```python
from build123d import *
from build123d.topology import SkipClean

# Parameters (mm, degrees)
BOSS_EXTRUDE1_DEPTH = 6
BOSS_EXTRUDE2_START = 6
SKETCH3_R           = 13
BOSS_EXTRUDE2_DEPTH = 8
BOSS_EXTRUDE3_START = -24
SKETCH4_R           = 9
BOSS_EXTRUDE3_DEPTH = 24
SKETCH5_R           = 10
SKETCH5_R_2         = 3
CUT_EXTRUDE1_DEPTH  = 30


with BuildPart() as part:
    # Sketch2 → Boss-Extrude1 (new body)
    with BuildSketch(Plane(origin=(0, 0, 0), x_dir=(0, 1, 0), z_dir=(0, 0, 1))):
        with BuildLine():
            Line((1.368421053, 12.927777219), (38.947368421, 8.949999613))
            ThreePointArc((38.947368421, 8.949999613), (47, 0), (38.947368421, -8.949999613))
            Line((38.947368421, -8.949999613), (1.368421053, -12.927777219))
            ThreePointArc((1.368421053, -12.927777219), (-13, 0), (1.368421053, 12.927777219))
        make_face()
    extrude(amount=BOSS_EXTRUDE1_DEPTH)

    # Sketch3 → Boss-Extrude2 (add)
    with SkipClean():  # the faces are left unmerged after this step: merging them gives an invalid solid
        with BuildSketch(Plane(origin=(0, 0, 0), x_dir=(0, 1, 0), z_dir=(0, 0, 1)).offset(BOSS_EXTRUDE2_START)):
            with Locations(Location((0, 0, 0), (0, 0, 83.957671581))):
                Circle(SKETCH3_R)
        extrude(amount=BOSS_EXTRUDE2_DEPTH)

    # Sketch4 → Boss-Extrude3 (add)
    with SkipClean():  # the faces are left unmerged after this step: merging them gives an invalid solid
        with BuildSketch(Plane(origin=(0, 0, 0), x_dir=(0, 1, 0), z_dir=(0, 0, 1)).offset(BOSS_EXTRUDE3_START)):
            with Locations(Location((38, 0, 0), (0, 0, 83.957671581))):
                Circle(SKETCH4_R)
        extrude(amount=BOSS_EXTRUDE3_DEPTH)

    # Sketch5 → Cut-Extrude1 (cut, symmetric)
    with SkipClean():  # the faces are left unmerged after this step: merging them gives an invalid solid
        with BuildSketch(Plane(origin=(0, 0, 0), x_dir=(0, 1, 0), z_dir=(0, 0, 1))):
            with Locations(Location((0, 0, 0), (0, 0, 270))):
                Circle(SKETCH5_R)
            with Locations(Location((38, 0, 0), (0, 0, 270))):
                Circle(SKETCH5_R_2)
        extrude(amount=CUT_EXTRUDE1_DEPTH, both=True, mode=Mode.SUBTRACT)


solid = part.part
```
Check sheet for the modelled part. Datum: model origin and axes. Units: mm. Coordinates: 2 decimals unless noted, no trailing zeros. Write each loop counter-clockwise with the first axis right and the second up, starting at its lowest first coordinate (ties: lowest second). Pieces come first, ordered by that corner, then holes. Notation, with made-up numbers: (-10, 82) - (21, 82) arc R20 cw to (21, 107) - close; hole circle Ø1 at (53.5, 20.5). An arc over 180 degrees is marked (long way). One line per question, with ' | ' between items.
Item 1: Sectioned sample at C-C on x = 7.5. Record the boundary of the cut face in (y, z), plus the area to 3 significant figures.
Determined:
outline: (-10.62, 0) - (-6.61, 0) - (-6.61, 14) - (-10.62, 14) - close; (6.61, 0) - (33.03, 0) - (33.03, -24) - (42.97, -24) - (42.97, 6) - (10.62, 6) - (10.62, 14) - (6.61, 14) - close | area: 545 mm2
Item 2: Gauge pin test, flat ends, axial feed: P1, Ø3, axis at x = 8, y = 36, coming from the +Z side; P2, Ø12, axis at y = 24, z = 4.5, coming from the +X side; P3, Ø10, axis at y = 40, z = 4.5, coming from the +X side; P4, Ø3, axis at y = 27, z = -15, coming from the -X side. Record the tip position at first contact, or that the pin passes through.
Determined:
P1: stops at z = 6 | P2: stops at x = 11.17 | P3: stops at x = 9.37 | P4: passes through
Item 3: Thickness scan on line 1 (Y direction, x = 0, z = -14.5); line 2 (X direction, y = 0, z = 9). Record the ranges inside material, lowest first. Write a range as [from, to].
Determined:
line 1: y = [29, 35], [41, 47] | line 2: x = [-13, -10], [10, 13]
Item 4: Sectioned sample at A-A on x = 0. Record the boundary of the cut face in (y, z).
Determined:
outline: (-13, 0) - (-10, 0) - (-10, 14) - (-13, 14) - close; (10, 0) - (29, 0) - (29, -24) - (35, -24) - (35, 6) - (13, 6) - (13, 14) - (10, 14) - close; (41, -24) - (47, -24) - (47, 6) - (41, 6) - close
Item 5: Sectioned sample at B-B on y = 0. Record the boundary of the cut face in (x, z).
Determined:
outline: (-13, 0) - (-10, 0) - (-10, 14) - (-13, 14) - close; (10, 0) - (13, 0) - (13, 14) - (10, 14) - close
Item 6: Sectioned sample at D-D on z = -10. Record the boundary of the cut face in (x, y), plus the area to 3 significant figures.
Determined:
outline: circle Ø18 at (0, 38); hole circle Ø6 at (0, 38) | area: 226 mm2
Item 7: Mould release check, pull along X, two halves, no side actions. Record for faces 1 (the face through (-2.17, -9.76, 6.9)), 2 (the face through (10.91, 20.42, 2.96)), 3 (the face through (-10.967, 19.895, 2.958)), 4 (the face through (0, 13, 0)): pulls with the +X half, pulls with the -X half, needs draft (parallel to the pull), parting line crosses it, or undercut.
Determined:
face 1: undercut | face 2: pulls with the +X half | face 3: pulls with the -X half | face 4: needs draft
